```python
from build123d import *

# Parameters (mm, degrees)
F1_DEPTH = 1.5
F2_R     = 1
F3_W     = 24
F3_H     = 11
F4_DEPTH = 1
F5_R     = 0.99999
F6_W     = 2
F6_H     = 5
F6_W_2   = 1
F6_W_3   = 5
F6_H_2   = 0.5
F7_DEPTH = 2


# Not quite as in the source:
# - a fillet or chamfer is up to 0.001 mm smaller than in the source, because OpenCascade refuses the exact size


with BuildPart() as f1:
    # F0 (on Top) → F1 (new body)
    with BuildSketch(Plane.XY):
        with BuildLine():
            ThreePointArc((0, 1), (0.2928932188, 0.2928932188), (1, 0))
            Line((1, 0), (26, 0))
            ThreePointArc((26, 0), (26.7071067812, 0.2928932188), (27, 1))
            Line((27, 1), (27, 11))
            ThreePointArc((27, 11), (26.7071067812, 11.7071067812), (26, 12))
            Line((26, 12), (1, 12))
            ThreePointArc((1, 12), (0.2928932188, 11.7071067812), (0, 11))
            Line((0, 11), (0, 1))
        make_face()
    extrude(amount=F1_DEPTH)

    # F2
    f2_edges = [f1.edges().sort_by_distance(p)[0] for p in [
        (0, 6, 1.5),
        (0.292893, 0.292893, 1.5),
        (13.5, 0, 1.5),
        (26.707107, 0.292893, 1.5),
        (27, 6, 1.5),
        (26.707107, 11.707107, 1.5),
        (13.5, 12, 1.5),
        (0.292893, 11.707107, 1.5),
    ]]
    fillet(f2_edges, radius=F2_R)

    # F3 (on Top) → F4 (cut)
    with BuildSketch(Plane.XY):
        with Locations((14, 6)):
            Rectangle(F3_W, F3_H)
    extrude(amount=F4_DEPTH, mode=Mode.SUBTRACT)

    # F5 (radius 1 in the source; OpenCascade refuses exactly that, so slightly less here)
    f5_edges = [f1.edges().sort_by_distance(p)[0] for p in [
        (14, 11.5, 1),
        (2, 6, 1),
        (14, 0.5, 1),
        (26, 6, 1),
    ]]
    fillet(f5_edges, radius=F5_R)

    # F6 (on face) → F7 (join)
    with BuildSketch(Plane(origin=(0, 0, 0), x_dir=(1, 0, 0), z_dir=(0, 0, -1))):
        with Locations((1, -6)):
            Rectangle(F6_W, F6_H)
        with Locations((26.5, -6)):
            Rectangle(F6_W_2, F6_H)
        with Locations((8.5, -0.25)):
            Rectangle(F6_W_3, F6_H_2)
        with Locations((18.5, -0.25)):
            Rectangle(F6_W_3, F6_H_2)
        with Locations((18.5, -11.75)):
            Rectangle(F6_W_3, F6_H_2)
    extrude(amount=F7_DEPTH)


solid = f1.part
```
Part model, mm, in its own coordinate system. A direction names the side the tool comes from. Round coordinates to 2 decimals unless told otherwise and drop trailing zeros. Loops run counter-clockwise (first coordinate to the right, second up) from the corner with the lowest first, then second, coordinate; pieces in that order, holes last.
Item 1: Cut at B-B, the plane y = 4.5. Give the cut face in (x, z).
Item 2: Drill centre lines: line 1 (X direction, y = 5, z = -0.1); line 2 (Y direction, x = 13.75, z = 0.05); line 3 (Z direction, x = 11.25, y = 6.75). Where is each one in solid material? Low to high.
Item 3: Drop flat-ended pins along their axis: P1, Ø1, axis at x = 15.5, y = 4, coming from the -Z side; P2, Ø0.5, axis at x = 26.5, z = -1, coming from the -Y side; P3, Ø0.6, axis at y = 0, z = -1, coming from the -X side. Give the stop position or say it passes through.
Item 4: Mould opens along X. For faces 4 (the face through (25.715, 6.077, 0.699)), 5 (the face through (26.699, 0.285, 0.247)), 6 (the face through (1, 8.5, -1)), 7 (the face through (14.168, 0.785, 0.699)) say: +X half, -X half, draft (parallel to the pull), parting line (faces both ways), or undercut.
Item 5: Cut at A-A, the plane z = -1.75. Give the cut face in (x, y).
Item 6: 3-axis set-ups, long thin cutter, end or side, ignore diameter. For faces 1 (the face through (26.5, 3.5, -1)), 2 (the face through (17, 0.5, -1)), 3 (the face through (14.168, 11.215, 0.699)): which of +Z, -Z, +X, -X, +Y, -Y reach the whole face in a straight line?
A:
1. outline: (0, -2) - (2, -2) - (2, 0) arc R1 cw to (3, 1) - (25, 1) arc R1 cw to (26, 0) - (26, -2) - (27, -2) - (27, 0.5) arc R1 ccw to (26, 1.5) - (1, 1.5) arc R1 ccw to (0, 0.5) - close
2. line 1: x = 0 to 2, 26 to 27
2. line 2: y = 0 to 0.5, 11.5 to 12
2. line 3: z = 1 to 1.5
3. P1: stops at z = 1
3. P2: stops at y = 3.5
3. P3: stops at x = 6
4. face 4: undercut
4. face 5: +X half
4. face 6: draft
4. face 7: undercut
5. outline: (0, 3.5) - (2, 3.5) - (2, 8.5) - (0, 8.5) - close; (6, 0) - (11, 0) - (11, 0.5) - (6, 0.5) - close; (16, 0) - (21, 0) - (21, 0.5) - (16, 0.5) - close; (16, 11.5) - (21, 11.5) - (21, 12) - (16, 12) - close; (26, 3.5) - (27, 3.5) - (27, 8.5) - (26, 8.5) - close
6. face 1: -Z, +X, -X, -Y
6. face 2: -Z, +X, -X
6. face 3: -Z
